Input: part model. Units: mm. Frame: model coordinates. Face numbers are marked on the shaded views. A direction names the side the tool comes from. Round coordinates to 2 decimals unless told otherwise and drop trailing zeros. Loops run counter-clockwise (first coordinate to the right, second up) from the corner with the lowest first, then second, coordinate; pieces in that order, holes last. Notation, with made-up numbers: (-38, 88.5) -> (19, 88.5) arc R32 cw to (19, 120.5) -> close; hole circle Ø7 at (36, 78). An arc over 180 degrees is marked (long way). Answer in a Markdown table with one row per item. Add a question column.
Q1. Pin query (flat end, axial travel): pin 1 (8 mm diameter, centred on y = -15.5, z = 11.5, fed in from -X); pin 2 (5 mm diameter, centred on x = 26.5, y = -3.5, fed in from +Z); pin 3 (9 mm diameter, centred on x = 51, z = 8.5, fed in from +Y); pin 4 (2 mm diameter, centred on y = 19.5, z = 10, fed in from +X). Return the tip coordinate at first contact, or that it passes through.
Q2. Section A-A, the plane z = 10. Output: boundary loops of the cut face in (x, y), and give its area (3 significant figures).
Q3. Section D-D, the plane x = -60. Output: boundary loops of the cut face in (y, z), and give its area (3 significant figures).
Q4. Mould query, pull axis Y, two halves, no side actions, for the marked faces 1, 2, 3 and 4. Classes: pulls with the +Y half, pulls with the -Y half, needs draft (parallel to the pull), parting line crosses it, or undercut.
Q5. Section C-C, the plane y = -34. Output: boundary loops of the cut face in (x, z), and give its area (3 significant figures).
Q6. Section B-B, the plane x = 0. Output: boundary loops of the cut face in (y, z), and give its area (3 significant figures).
Q7. Ray query, L1, parallel to Y at x = 0, z = 17; L2, parallel to X at y = -32.25, z = 10; L3, parallel to Y at x = 0, z = 5. Return the intervals inside material, ascending. Write a range as from..to.
Q8. Reachability of the marked faces 5, 6 and 7 from +Z, -Z, +X, -X, +Y, -Y: full face, straight path, thin tool, end or side. Return the list, or none.
Autodesk Inventor part; units mm, degrees
ref_plane "YZ Plane" through (0, 0, 0) normal (1, 0, 0) x (0, 1, 0)
ref_plane "XZ Plane" through (0, 0, 0) normal (0, 1, 0) x (-1, 0, 0)
ref_plane "XY Plane" through (0, 0, 0) normal (0, 0, 1) x (1, 0, 0)
sketch "Sketch6" plane through (0, 0, 0) normal (0, 0, 1) x (1, 0, 0)
  circle A0 centre (0, 0) radius 17.07
  circle A1 centre (0, 0) radius 28.07
  line L0 (-40, -40) -> (40, -40)
  line L1 (40, -40) -> (40, 0)
  line L2 (-40, 0) -> (-40, -40)
  circle A2 centre (0, 0) radius 40
  line L3 (-40, -40) -> (-80, -40)
  line L4 (-80, -40) -> (-80, -20)
  line L5 (-80, -20) -> (-40, -20)
  line L6 (-40, -20) -> (-40, -40)
  line L7 (40, -40) -> (80, -40)
  line L8 (80, -40) -> (80, -20)
  line L9 (80, -20) -> (40, -20)
  line L10 (40, -20) -> (40, -40)
  dimension "d29" = 34.14
  dimension "d30" = 56.14
extrude "Extrusion5" add sketch "Sketch6" along normal blind 20 contours L2 A2 L0 | L3 L4 L5 L2 | A2 L1 L0 | A2 | L1 L9 L8 L7
sketch "Sketch7" plane through (0, 0, 0) normal (0, 0, -1) x (-1, 0, 0)
  circle A0 centre (0, 0) radius 17.07
  circle A1 centre (0, 0) radius 28.07
  dimension "d39" = 34.14
  dimension "d40" = 56.14
extrude "Extrusion6" add sketch "Sketch7" against normal blind 8
sketch "Sketch8" plane through (-80, -20, 0) normal (0, 1, 0) x (1, 0, 0)
  line L0 (0, 0) -> (0, -20)
  line L1 (0, -20) -> (160, -20)
  line L2 (0, 0) -> (40, 0)
  line L3 (40, 0) -> (40, -20)
  line L4 (40, -20) -> (0, -20)
  line L5 (0, -20) -> (0, 0)
  circle A0 centre (20, -10) radius 6
  point P0 (80, 0)
  dimension "d44" = 12
extrude "Extrusion7" cut sketch "Sketch8" against normal blind 20 contours A0
thread "Thread3"
sketch "Sketch9" plane through (40, -20, 0) normal (0, 1, 0) x (1, 0, 0)
  line L0 (0, 0) -> (0, -20)
  line L1 (40, 0) -> (40, -20)
  line L2 (0, 0) -> (40, 0)
  line L3 (40, 0) -> (40, -20)
  line L4 (40, -20) -> (0, -20)
  line L5 (0, -20) -> (0, 0)
  circle A0 centre (20, -10) radius 6
  point P0 (-40, 0)
  dimension "d49" = 12
extrude "Extrusion8" cut sketch "Sketch9" against normal blind 20 contours A0
thread "Thread4"
fillet "Fillet3" radius 1 15 edges at (-60, -20, 20) (-60, -20, 0) (-80, -20, 10) (-80, -30, 0) (-80, -30, 20) (60, -20, 20) (60, -20, 0) (80, -30, 20) (80, -30, 0) (0, 40, 20) (-40, -10, 20) (40, -10, 20) (0, 40, 0) (-40, -10, 0) (40, -10, 0)
properties part number "Chumacera (pieza extra)"
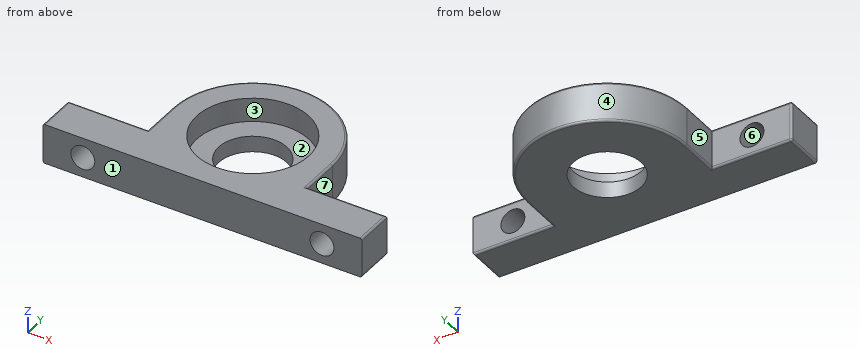
Answer block:
| question | item | result |
|---|---|---|
| 1 | pin 1 | x = -40 |
| 1 | pin 2 | z = 20 |
| 1 | pin 3 | y = -20 |
| 1 | pin 4 | x = 35.46 |
| 2 | outline | (-80, -40) -> (-66, -40) -> (-66, -20) -> (-79, -20) arc R1 ccw to (-80, -21) -> close; (-54, -40) -> (54, -40) -> (54, -20) -> (40, -20) -> (40, 0) arc R40 ccw to (-40, 0) -> (-40, -20) -> (-54, -20) -> close; (66, -40) -> (80, -40) -> (80, -20) -> (66, -20) -> close; hole circle Ø56.14 at (0, 0) |
| 2 | area | 4,360 mm^2 |
| 3 | outline | (-40, 0) -> (-21, 0) arc R1 ccw to (-20, 1) -> (-20, 4) -> (-40, 4) -> close; (-40, 16) -> (-20, 16) -> (-20, 19) arc R1 ccw to (-21, 20) -> (-40, 20) -> close |
| 3 | area | 160 mm^2 |
| 4 | face 1 | pulls with the -Y half |
| 4 | face 2 | undercut |
| 4 | face 3 | undercut |
| 4 | face 4 | pulls with the +Y half |
| 5 | outline | (-80, 1) arc R1 ccw to (-79, 0) -> (79, 0) arc R1 ccw to (80, 1) -> (80, 19) arc R1 ccw to (79, 20) -> (-79, 20) arc R1 ccw to (-80, 19) -> close; hole circle Ø12 at (-60, 10); hole circle Ø12 at (60, 10) |
| 5 | area | 2,970 mm^2 |
| 6 | outline | (-40, 0) -> (-17.07, 0) -> (-17.07, 8) -> (-28.07, 8) -> (-28.07, 20) -> (-40, 20) -> close; (17.07, 0) -> (39, 0) arc R1 ccw to (40, 1) -> (40, 19) arc R1 ccw to (39, 20) -> (28.07, 20) -> (28.07, 8) -> (17.07, 8) -> close |
| 6 | area | 653 mm^2 |
| 7 | L1 | -40..-28.07, 28.07..40 |
| 7 | L2 | -80..-66, -54..54, 66..80 |
| 7 | L3 | -40..-17.07, 17.07..40 |
| 8 | face 5 | +Z, -Z, -X, +Y |
| 8 | face 6 | +Y, -Y |
| 8 | face 7 | +Z, -Z, +X, +Y |
